Autodesk Inventor part; units mm, degrees
ref_plane "YZ Plane" through (0, 0, 0) normal (1, 0, 0) x (0, 1, 0)
ref_plane "XZ Plane" through (0, 0, 0) normal (0, 1, 0) x (-1, 0, 0)
ref_plane "XY Plane" through (0, 0, 0) normal (0, 0, 1) x (1, 0, 0)
sketch "Skizze1" plane through (0, 0, 0) normal (0, 1, 0) x (-1, 0, 0)
  line L0 (0, 0) -> (23.3, 0)
  line L1 (23.3, 0) -> (23.3, 26.8)
  line L2 (23.3, 26.8) -> (0, 26.8)
  line L3 (0, 26.8) -> (0, 0)
  dimension "d0" = 23.3
  dimension "d1" = 26.8
extrude "Extrusion1" add sketch "Skizze1" along normal blind 0.4
sketch "Skizze2" plane through (0, 0, 0) normal (0, -1, 0) x (1, 0, 0)
  line L0 (0, 0) -> (-23.3, 0)
  line L1 (0, 26.8) -> (0, 0)
  line L2 (-23.3, 26.8) -> (0, 26.8)
  line L3 (-23.3, 0) -> (-23.3, 26.8)
  line L4 (-17.8, 3) -> (-5.5, 3)
  line L5 (-5.5, 3) -> (-5.5, 9.8)
  line L6 (-5.5, 9.8) -> (-17.8, 9.8)
  line L7 (-17.8, 9.8) -> (-17.8, 3)
  dimension "d4" = 3
  dimension "d5" = 17
  dimension "d6" = 5.5
  dimension "d7" = 5.5
extrude "Extrusion2" add sketch "Skizze2" along normal blind 1 contours L7 L6 L5 L4
sketch "Skizze3" plane through (0, -1, 0) normal (0, -1, 0) x (1, 0, 0)
  line L0 (-17.8, 3) -> (-5.5, 3)
  line L1 (-5.5, 3) -> (-5.5, 9.8)
  line L2 (-5.5, 9.8) -> (-17.8, 9.8)
  line L3 (-17.8, 9.8) -> (-17.8, 3)
  circle A0 centre (-11.65, 6.4) radius 2.9125
  point P0 (0, 0)
extrude "Extrusion3" cut sketch "Skizze3" against normal blind 1 contours A0
ref_plane "Work Plane1" through (-11.65, 0, 0) normal (-1, 0, 0) x (0, 0, 1)
sketch "Sketch5" plane through (0, 0, 26.8) normal (1, 0, 0) x (0, 0, -1)
  line L0 (23.3125, -1) -> (23.3125, 0)
  line L1 (17.4875, -1) -> (17.4875, 0)
  circle A0 centre (20.4499, -0.5) radius 0.5025
  point P0 (26.8, 0)
extrude "Extrusion5" cut sketch "Sketch5" against normal through all
ref_plane "Work Plane3" through (-52.1328, -19.1011, -24.6499) normal (0, 1, 0) x (1, 0, 0)
sketch "Sketch6" plane through (-52.1328, -19.1011, -24.6499) normal (0, 1, 0) x (1, 0, 0)
  line L0 (46.6328, -31.0499) -> (52.1328, -31.0499) construction
  line L1 (52.1328, -51.4499) -> (52.1328, -31.0499) construction
  line L2 (28.8328, -51.4499) -> (52.1328, -51.4499) construction
  line L3 (28.8328, -31.0499) -> (28.8328, -51.4499) construction
  line L4 (28.8328, -31.0499) -> (34.3328, -31.0499) construction
  line L5 (34.3328, -31.0499) -> (34.3328, -34.4499) construction
  line L6 (34.3328, -34.4499) -> (46.6328, -34.4499) construction
  line L7 (46.6328, -34.4499) -> (46.6328, -31.0499) construction
  line L8 (6.9828, -36.0499) -> (6.9828, 22.8301) construction
  line L9 (46.6328, -31.5025) -> (34.3328, -31.5025) construction
  line L10 (-16.7355, -31.5025) -> (-33.6581, -41.2728) construction
  line L11 (-33.6581, -41.2728) -> (-33.6581, -21.7322) construction
  line L12 (-33.6581, -21.7322) -> (-16.7355, -31.5025) construction
  point P0 (52.1328, -24.6499)
  point P1 (-28.0172, -31.5025)
  dimension "d16" = 35
properties part number "02_Nanoscopy_Chip"
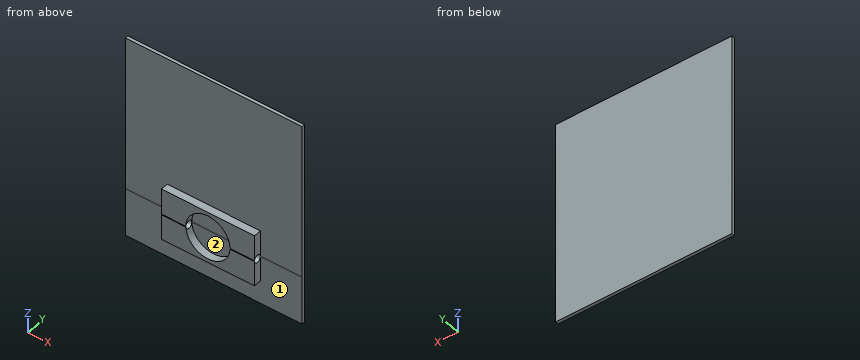
Geometry: final body of the model. Coordinates: model frame, mm. Face numbers are marked on the shaded views. Round coordinates to 2 decimals unless told otherwise and drop trailing zeros. Order: outer loops, then holes, each group sorted by start corner. A loop starts at its lowest first (then second) coordinate and runs counter-clockwise, first axis right, second up. Notation, with made-up numbers: M 21,87 L 26,87 A33 ccw 26,119 Z; hole C -26,66 d3. An arc over 180 degrees is marked long. Use one line per item in the form item = value. Start each with the question number.
Q1. Material intervals for line 1 (Y direction, x = -21.75, z = 4); line 2 (Z direction, x = -11.5, y = -0.7); line 3 (Z direction, x = -14.75, y = -0.5), sorted ascending. Write a range as [from, to].
Q2. Mould query, pull axis X, two halves, no side actions, for the marked faces 1 and 2. Classes: +X half, -X half, draft (parallel to the pull), parting line (faces both ways), or undercut.
Q3. Cut plane C-C (z = 4.5). Return loops of the section in (x, y), and give its area (3 significant figures).
Q4. Pin query (flat end, axial travel): pin 1 Ø10 at (x, z) = (-10, 18) entering from -Y; pin 2 Ø0.5 at (y, z) = (-0.5, 5) entering from -X; pin 3 Ø0.5 at (x, y) = (-9.5, -0.5) entering from +Z. Return the tip coordinate at first contact, or that it passes through.
Geometry results:
q1.line_1 = [0, 0.4]
q1.line_2 = [3, 3.49], [9.31, 9.8]
q1.line_3 = [3, 5.85], [6.85, 9.8]
q2.face_1 = draft
q2.face_2 = undercut
q3.outline = M -23.3,0 L -17.8,0 L -17.8,-1 L -13.86,-1 L -13.86,0 L -9.44,0 L -9.44,-1 L -5.5,-1 L -5.5,0 L 0,0 L 0,0.4 L -23.3,0.4 Z
q3.area = 17.2 mm^2
q4.pin_1 = 0
q4.pin_2 = -17.8
q4.pin_3 = 9.8
